Check sheet for the modelled part. Datum: model origin and axes. Units: mm. A direction names the side the tool comes from. Round coordinates to 2 decimals unless told otherwise and drop trailing zeros. Write each loop counter-clockwise with the first axis right and the second up, starting at its lowest first coordinate (ties: lowest second). Pieces come first, ordered by that corner, then holes. Notation, with made-up numbers: M 75,-33 L 123,-33 A23 ccw 123,5 Z; hole C -3,22.25 d6. An arc over 180 degrees is marked long. One line per item, written item: value.
from build123d import *

# Parameters (mm, degrees)
F0_R     = 225
F0_R_2   = 160
F1_DEPTH = 150
F2_R     = 50
F0_R_3   = 51.929068635
F3_DEPTH = 5


with BuildPart() as f1:
    # F0 (on Right) → F1 (new body, symmetric)
    with BuildSketch(Plane.YZ):
        Circle(F0_R)
        Circle(F0_R_2, mode=Mode.SUBTRACT)
    extrude(amount=F1_DEPTH, both=True)

    # F2
    f2_edges = [f1.edges().sort_by_distance(p)[0] for p in [
        (150, -225, 0),
        (-150, -225, 0),
        (0, 225, 0),
    ]]
    fillet(f2_edges, radius=F2_R)

    # F0 (on Right) → F3 (join)
    with BuildSketch(Plane.YZ):
        Circle(F0_R_2)
        with BuildLine():
            ThreePointArc((74.6640796825, 65.4801758986), (92.944153106, 34.982318876), (99.3095072515, 0))
            ThreePointArc((99.3095072515, 0), (92.944153106, -34.982318876), (74.6640796825, -65.4801758986))
            ThreePointArc((74.6640796825, -65.4801758986), (75.8536647795, -67.1491372402), (76.2737192458, -69.1551529202))
            ThreePointArc((76.2737192458, -69.1551529202), (73.1638044573, -73.7841461037), (67.7026880885, -72.6548295444))
            ThreePointArc((67.7026880885, -72.6548295444), (0, -99.3095072515), (-67.7026880885, -72.6548295444))
            ThreePointArc((-67.7026880885, -72.6548295444), (-74.8621832921, -72.6369521373), (-74.6640796825, -65.4801758986))
            ThreePointArc((-74.6640796825, -65.4801758986), (-99.3095072515, 0), (-74.6640796825, 65.4801758986))
            ThreePointArc((-74.6640796825, 65.4801758986), (-74.8621832921, 72.6369521373), (-67.7026880885, 72.6548295444))
            ThreePointArc((-67.7026880885, 72.6548295444), (0, 99.3095072515), (67.7026880885, 72.6548295444))
            ThreePointArc((67.7026880885, 72.6548295444), (73.1638044573, 73.7841461037), (76.2737192458, 69.1551529202))
            ThreePointArc((76.2737192458, 69.1551529202), (75.8536647795, 67.1491372402), (74.6640796825, 65.4801758986))
        make_face(mode=Mode.SUBTRACT)
        with BuildLine():
            ThreePointArc((-71.2737192458, 64.1551529202), (-73.0937624997, 64.4981750853), (-74.6640796825, 65.4801758986))
            ThreePointArc((-74.6640796825, 65.4801758986), (-99.3095072515, 0), (-74.6640796825, -65.4801758986))
            ThreePointArc((-74.6640796825, -65.4801758986), (-73.0937624997, -64.4981750853), (-71.2737192458, -64.1551529202))
            Line((-71.2737192458, -64.1551529202), (-71.2737192458, 64.1551529202))
        make_face()
        with BuildLine():
            ThreePointArc((66.2737192458, 69.1551529202), (66.6447260623, 71.0452381317), (67.7026880885, 72.6548295444))
            ThreePointArc((67.7026880885, 72.6548295444), (0, 99.3095072515), (-67.7026880885, 72.6548295444))
            ThreePointArc((-67.7026880885, 72.6548295444), (-66.6447260623, 71.0452381317), (-66.2737192458, 69.1551529202))
            Line((-66.2737192458, 69.1551529202), (66.2737192458, 69.1551529202))
        make_face()
        with BuildLine():
            ThreePointArc((-67.7026880885, -72.6548295444), (0, -99.3095072515), (67.7026880885, -72.6548295444))
            ThreePointArc((67.7026880885, -72.6548295444), (66.6447260623, -71.0452381317), (66.2737192458, -69.1551529202))
            Line((66.2737192458, -69.1551529202), (-66.2737192458, -69.1551529202))
            ThreePointArc((-66.2737192458, -69.1551529202), (-66.6447260623, -71.0452381317), (-67.7026880885, -72.6548295444))
        make_face()
        with BuildLine():
            Line((71.2737192458, -64.1551529202), (71.2737192458, 64.1551529202))
            ThreePointArc((71.2737192458, 64.1551529202), (67.7381853399, 65.6196190142), (66.2737192458, 69.1551529202))
            Line((66.2737192458, 69.1551529202), (-66.2737192458, 69.1551529202))
            ThreePointArc((-66.2737192458, 69.1551529202), (-67.7381853399, 65.6196190142), (-71.2737192458, 64.1551529202))
            Line((-71.2737192458, 64.1551529202), (-71.2737192458, -64.1551529202))
            ThreePointArc((-71.2737192458, -64.1551529202), (-67.7381853399, -65.6196190142), (-66.2737192458, -69.1551529202))
            Line((-66.2737192458, -69.1551529202), (66.2737192458, -69.1551529202))
            ThreePointArc((66.2737192458, -69.1551529202), (67.7381853399, -65.6196190142), (71.2737192458, -64.1551529202))
        make_face()
        Circle(F0_R_3, mode=Mode.SUBTRACT)
        with BuildLine():
            ThreePointArc((74.6640796825, -65.4801758986), (92.944153106, -34.982318876), (99.3095072515, 0))
            ThreePointArc((99.3095072515, 0), (92.944153106, 34.982318876), (74.6640796825, 65.4801758986))
            ThreePointArc((74.6640796825, 65.4801758986), (73.0937624997, 64.4981750853), (71.2737192458, 64.1551529202))
            Line((71.2737192458, 64.1551529202), (71.2737192458, -64.1551529202))
            ThreePointArc((71.2737192458, -64.1551529202), (73.0937624997, -64.4981750853), (74.6640796825, -65.4801758986))
        make_face()
    extrude(amount=F3_DEPTH)


solid = f1.part
Q1. Sectioned sample at A-A on z = 0. Enter the section's corners in (x, y), and give its area (3 significant figures).
Completed:
outline: M -150,-175 A50 ccw -100,-225 L 100,-225 A50 ccw 150,-175 L 150,-160 L 5,-160 L 5,-51.93 L 0,-51.93 L 0,-160 L -150,-160 Z; M -150,160 L 0,160 L 0,51.93 L 5,51.93 L 5,160 L 150,160 L 150,175 A50 ccw 100,225 L -100,225 A50 ccw -150,175 Z
area: 37,900 mm^2
Q2. Access from +Z, -Z, +X, -X, +Y, -Y to the whole of each face (thin tool, end or side, straight path). Record for faces 5 (the cylindrical face through (76.485, -34.685, -156.195)), 6 (the flat face through (-150, 77, -142)), 7 (the flat face through (0, -38, 38)).
Completed:
face 5: +X
face 6: +Z, -Z, -X, +Y, -Y
face 7: -X
Q3. Sectioned sample at C-C on x = -114. Enter the section's corners in (y, z).
Completed:
outline: C 0,0 d446; hole C 0,0 d320
Q4. Sectioned sample at D-D on x = 41.5. Enter the section's corners in (y, z), and give its area (3 significant figures).
Completed:
outline: C 0,0 d450; hole C 0,0 d320
area: 78,600 mm^2
Q5. Scan lines: line 1 (Z direction, x = 102, y = 0); line 2 (Z direction, x = -34, y = 0); line 3 (X direction, y = 22.5, z = 66.5). Record each from-to range of solid material in increasing order. Write a range as [from, to].
Completed:
line 1: [-224.96, -160], [160, 224.96]
line 2: [-225, -160], [160, 225]
line 3: [0, 5]
Q6. Depth check by flat-ended pin: P1, Ø1, axis at x = 74, z = -110.5, coming from the +Y side; P2, Ø1.5, axis at x = 43.5, z = 35.5, coming from the -Y side; P3, Ø2, axis at x = -106.5, y = 162, coming from the -Z side. Enter the tip coordinate at first touch or a pass-through.
Completed:
P1: y = 196.28
P2: y = -222.3
P3: z = -156.58
Q7. Draft check along Y on faces 1 (the cylindrical face through (2.465, -6.76, 51.487)), 2 (the cylindrical face through (1.4, -224.782, 9.893)), 3 (the cylindrical face through (-76.05, -34.685, -156.195)), 4 (the flat face through (150, 77, -142)). Enter one of: pulls with the +Y half, pulls with the -Y half, needs draft (parallel to the pull), parting line crosses it, or undercut.
Completed:
face 1: undercut
face 2: parting line crosses it
face 3: undercut
face 4: needs draft
